Can you work these out from the model? Positions are in its coordinate system, mm. A direction names the side the tool comes from. Give positions to 0.01 mm unless a question says otherwise; leave off trailing zeros. Order: outer loops, then holes, each group sorted by start corner. A loop starts at its lowest first (then second) coordinate and runs counter-clockwise, first axis right, second up. Notation, with made-up numbers: (-12, 50) - (33, 50) arc R38 ccw to (33, 89) - close; hole circle Ø5 at (43.25, 9.5). An arc over 180 degrees is marked (long way). One line per question, with ' | ' between items.
```python
from build123d import *

# Parameters (mm, degrees)
PAD_DEPTH          = 10
PAD001_DEPTH       = 70
PAD002_DEPTH       = 3
PAD002_DEPTH_BACK  = 3
POLARPATTERN_COUNT = 4
POCKET_DEPTH       = 70.001
POCKET_DEPTH_BACK  = 10.001


with BuildPart() as part:
    # Sketch → Pad (new body)
    with BuildSketch(Plane.XY):
        with BuildLine():
            ThreePointArc((50, 25), (0, 75), (-50, 25))
            Line((-50, 25), (-50, -25))
            ThreePointArc((-50, -25), (0, -75), (50, -25))
            Line((50, 25), (50, -25))
        make_face()
    extrude(amount=PAD_DEPTH)

    # Sketch001 (on Face6 of Pad) → Pad001 (join)
    with BuildSketch(Plane.XY.offset(10)):
        Polygon((-17.5, 17.5), (17.5, 17.5), (17.5, 18), (18.5, 18), (18.5, -18), (17.5, -18), (17.5, -17.5), (-17.5, -17.5), align=None)
        Polygon((-14.5, 15), (-14.5, -15), (14.5, -15), (14.5, -15.5), (15.5, -15.5), (15.5, 15.5), (14.5, 15.5), (14.5, 15), align=None, mode=Mode.SUBTRACT)
    extrude(amount=PAD001_DEPTH)

    # Sketch002 → Pad002 (join, two sides)
    with BuildSketch(Plane.YZ) as pad002_sk:
        Polygon((17, 50), (37, 10), (17, 10), align=None)
    pad002 = extrude(amount=PAD002_DEPTH) + extrude(pad002_sk.sketch, amount=-PAD002_DEPTH_BACK)

    # PolarPattern: Pad002 ×4 about axis
    polarpattern_axis = Axis((0, 0, 0), (0, 0, 1))
    for i in range(1, POLARPATTERN_COUNT):
        add(pad002.rotate(polarpattern_axis, i * 360 / POLARPATTERN_COUNT))

    # Sketch003 (on Face5 of Pad001) → Pocket (cut, two sides)
    with BuildSketch(Plane.XY.offset(10)) as pocket_sk:
        Polygon((20, 45), (10, 62.320508), (-10, 62.320508), (-20, 45), (-10, 27.679492), (10, 27.679492), align=None)
        Polygon((-26, 17.875644), (-19, 30), (-26, 42.124356), (-40, 42.124356), (-47, 30), (-40, 17.875644), align=None)
        Polygon((40, 17.875644), (47, 30), (40, 42.124356), (26, 42.124356), (19, 30), (26, 17.875644), align=None)
        Polygon((-19, 0), (-26, 12.124356), (-40, 12.124356), (-47, 0), (-40, -12.124356), (-26, -12.124356), align=None)
        Polygon((20, -45), (10, -27.679492), (-10, -27.679492), (-20, -45), (-10, -62.320508), (10, -62.320508), align=None)
        Polygon((40, -12.124356), (47, 0), (40, 12.124356), (26, 12.124356), (19, 0), (26, -12.124356), align=None)
        Polygon((40, -42.124356), (47, -30), (40, -17.875644), (26, -17.875644), (19, -30), (26, -42.124356), align=None)
        Polygon((-19, -30), (-26, -17.875644), (-40, -17.875644), (-47, -30), (-40, -42.124356), (-26, -42.124356), align=None)
    extrude(amount=POCKET_DEPTH, mode=Mode.SUBTRACT)
    extrude(pocket_sk.sketch, amount=-POCKET_DEPTH_BACK, mode=Mode.SUBTRACT)


solid = part.part
```
(1) Imagine slicing it at C-C (y = 5.5). List the corners of the cut face in (x, z) for me.
Answer below:
outline: (-50, 0) - (-43.82, 0) - (-43.82, 10) - (-50, 10) - close; (-22.18, 0) - (22.18, 0) - (22.18, 10) - (18.5, 10) - (18.5, 80) - (15.5, 80) - (15.5, 10) - (-14.5, 10) - (-14.5, 80) - (-17.5, 80) - (-17.5, 10) - (-22.18, 10) - close; (43.82, 0) - (50, 0) - (50, 10) - (43.82, 10) - close
(2) Imagine slicing it at A-A (x = 0). List the corners of the cut face in (y, z) for me, and give its area (3 significant figures).
Answer below:
outline: (-75, 0) - (-62.32, 0) - (-62.32, 10) - (-75, 10) - close; (-27.68, 0) - (27.68, 0) - (27.68, 28.64) - (17.5, 49) - (17.5, 80) - (15, 80) - (15, 10) - (-15, 10) - (-15, 80) - (-17.5, 80) - (-17.5, 49) - (-27.68, 28.64) - close; (62.32, 0) - (75, 0) - (75, 10) - (62.32, 10) - close | area: 1,740 mm^2
(3) If we mould it in two halves opening along X, with no side actions, what happens to faces 1 (the face through (22.451, 24.023, 5.07)), 2 (the face through (-1.099, -74.988, 4.93)), 3 (the face through (-3, -22, 25)), 4 (the face through (33, -12.124, 5))? For each: released by +X, released by -X, zero draft, split by the parting line, or undercut.
Answer below:
face 1: undercut | face 2: split by the parting line | face 3: released by -X | face 4: undercut
(4) If I drill on line 1 (X direction, y = 4, z = 45.5); line 2 (Y direction, x = 44, z = 8.5); line 3 (Y direction, x = 13.5, z = 4.5), over which ranges is the centre line in solid material (lowest first)?
Answer below:
line 1: -17.5 to -14.5, 15.5 to 18.5 | line 2: -48.75 to -35.2, -24.8 to -5.2, 5.2 to 24.8, 35.2 to 48.75 | line 3: -73.14 to -56.26, -33.74 to 33.74, 56.26 to 73.14
(5) Will these pins go through, and if not, where does the flat tip stop? pin 1 (11 mm diameter, centred on y = 22.5, z = 20.5, fed in from +X); pin 2 (11 mm diameter, centred on x = -34, z = 7, fed in from -Y); pin 3 (11 mm diameter, centred on x = 32.5, z = 7, fed in from +Y).
Answer below:
pin 1: x = 18.5 | pin 2: y = -66.08 | pin 3: y = 67.08
(6) On a 3-axis mill with a long thin cutter (end or side, diameter ignored), from which of +Z, -Z, +X, -X, +Y, -Y can I reach the whole of each face in a straight line? I mean faces 5 (the face through (20.22, 2.11, 12.46)), 6 (the face through (19, 1, 46)), 7 (the face through (0, -15, 45)). Say none if no direction works.
Answer below:
face 5: +Z, -Z | face 6: +Z, +X, +Y, -Y | face 7: +Z
